Can you work these out from the model? Positions are in its coordinate system, mm. Coordinates: 2 decimals unless noted, no trailing zeros. Write each loop counter-clockwise with the first axis right and the second up, starting at its lowest first coordinate (ties: lowest second). Pieces come first, ordered by that corner, then holes. Notation, with made-up numbers: (78.25, -23.75) -> (91.25, -23.75) arc R22 cw to (91.25, -7.75) -> close; hole circle Ø10 at (42.5, 51). An arc over 180 degrees is marked (long way). Use one line per item in the form item = value.
```python
from build123d import *

# Parameters (mm, degrees)
ESTRUSIONE_ESTRUSIONE1_DEPTH = 39
FORO_PER_VITE_M8_1_D         = 9
FORO_PER_VITE_M8_1_DEPTH     = 30
FORO_PER_VITE_M8_1_TIP       = 2.703872786
RACCORDO1_R                  = 1.5


with BuildPart() as part:
    # Schizzo1 → Estrusione-Estrusione1 (new body)
    with BuildSketch(Plane.XY):
        with BuildLine():
            Line((-7.75, 15), (-21.5, 15))
            Line((-21.5, 15), (-22.5, 0))
            Line((-22.5, 0), (22.5, 0))
            Line((22.5, 0), (21.5, 15))
            Line((21.5, 15), (7.75, 15))
            ThreePointArc((7.75, 15), (0, 7.25), (-7.75, 15))
        make_face()
    extrude(amount=ESTRUSIONE_ESTRUSIONE1_DEPTH)

    # Foro per Vite M8-1
    with Locations(Plane(origin=(0, 0, 0), x_dir=(-1, 0, 0), z_dir=(0, -1, 0))):
        with Locations((-15.5, -7.5), (15.5, -7.5), (15.5, -31.5), (-15.5, -31.5)):
            Hole(FORO_PER_VITE_M8_1_D / 2, depth=FORO_PER_VITE_M8_1_DEPTH)
            with Locations((0, 0, -(FORO_PER_VITE_M8_1_DEPTH + FORO_PER_VITE_M8_1_TIP / 2))):  # 118° drill point
                Cone(0, FORO_PER_VITE_M8_1_D / 2, FORO_PER_VITE_M8_1_TIP, mode=Mode.SUBTRACT)

    # Raccordo1
    raccordo1_edges = [part.edges().sort_by_distance(p)[0] for p in [
        (-22, 7.5, 39),
        (22, 7.5, 39),
        (22, 7.5, 0),
        (-22, 7.5, 0),
    ]]
    fillet(raccordo1_edges, radius=RACCORDO1_R)


solid = part.part
```
Q1. Will these pins go through, and if not, where does the flat tip stop? pin 1 (4 mm diameter, centred on y = 6.5, z = 11.5, fed in from +X); pin 2 (1.5 mm diameter, centred on y = 6, z = 29.5, fed in from +X); pin 3 (1 mm diameter, centred on x = -6.5, z = 27.5, fed in from +Y).
Return value:
pin_1 = 22.2
pin_2 = 22.15
pin_3 = 11.67
Q2. If I drill on line 1 (Z direction, x = 15.5, y = 12); line 2 (Z direction, x = 18.5, y = 4.25); line 3 (X direction, y = 11, z = 31.5), over which ranges is the centre line in solid material (lowest first)? Write a range as from..to.
Return value:
line_1 = 0..3, 12..27, 36..39
line_2 = 0..4.15, 10.85..28.15, 34.85..39
line_3 = -21.77..-20, -11..-6.64, 6.64..11, 20..21.77
Q3. Suppose I cut it at A-A (x = -15.5). Write out the boundary of the cut face in (y, z), then the cut area to 3 significant figures.
Return value:
outline = (0, 0) -> (15, 0) -> (15, 3) -> (0, 3) -> close; (0, 12) -> (15, 12) -> (15, 27) -> (0, 27) -> close; (0, 36) -> (15, 36) -> (15, 39) -> (0, 39) -> close
area = 315 mm2
Q4. Suppose I cut it at D-D (x = 0). Write out the boundary of the cut face in (y, z), then the cut area to 3 significant figures.
Return value:
outline = (0, 0) -> (7.25, 0) -> (7.25, 39) -> (0, 39) -> close
area = 283 mm2
Q5. Thinking about a two-plate mould opening in Z: for faces 1 (the cylindrical face through (21.54, 7.63, 0.43)), 2 (the cylindrical face through (21.54, 7.63, 38.57)), 3 (the flat face through (15, 15, 19)), 4 (the cylindrical face through (11.9, 7.6, 10.2)), which applies, released by +Z, released by -Z, zero draft, split by the parting line, or undercut?
Return value:
face_1 = released by -Z
face_2 = released by +Z
face_3 = zero draft
face_4 = undercut
Q6. Suppose I cut it at B-B (z = 7.5). Write out the boundary of the cut face in (x, y), then the cut area to 3 significant figures.
Return value:
outline = (-22.5, 0) -> (-20, 0) -> (-20, 15) -> (-21.5, 15) -> close; (-11, 0) -> (11, 0) -> (11, 15) -> (7.75, 15) arc R7.75 cw to (-7.75, 15) -> (-11, 15) -> close; (20, 0) -> (22.5, 0) -> (21.5, 15) -> (20, 15) -> close
area = 296 mm2
Q7. Suppose I cut it at C-C (y = 13.25). Give the number of separate pieces and of enclosed holes in the cut face, then the cut area to 3 significant figures.
Return value:
separate_pieces = 2
enclosed_holes = 4
area = 841 mm2
